from build123d import *

# Parameters (mm, degrees)
BASE_DEPTH            = 7.5
MOUNT_START           = -2
MOUNT_DEPTH           = 4
MOUNT_HOLE_DEPTH      = 204.131478566
MOUNT_HOLE_DEPTH_BACK = 204.131478566
SKETCH12_R            = 1.5
SKETCH14_R            = 1.5
SHAFT_HOLE_DEPTH      = 37.394984425
SKETCH13_W            = 2.5
SKETCH13_H            = 3


with BuildPart() as part:
    # Sketch9 → base (new, symmetric)
    with BuildSketch(Plane(origin=(0, 0, 0), x_dir=(1, 0, 0), z_dir=(0, 1, 0))):
        with BuildLine():
            ThreePointArc((-187.113473072, -32.993153757), (-190, 0), (-187.113473072, 32.993153757))
            Line((-187.113473072, 32.993153757), (-196.961550602, 34.729635533))
            ThreePointArc((-196.961550602, 34.729635533), (-200, 0), (-196.961550602, -34.729635533))
            Line((-196.961550602, -34.729635533), (-187.113473072, -32.993153757))
        make_face()
    extrude(amount=BASE_DEPTH, both=True)

    # Sketch11 → mount (cut)
    with BuildSketch(Plane(origin=(0, 0, 0), x_dir=(1, 0, 0), z_dir=(0, 1, 0)).offset(MOUNT_START)):
        with BuildLine():
            Line((-189.73665961, -10), (-199.749843554, -10))
            ThreePointArc((-199.749843554, -10), (-198.7407137, -22.408228804), (-196.961550602, -34.729635533))
            Line((-196.961550602, -34.729635533), (-187.113473072, -32.993153757))
            ThreePointArc((-187.113473072, -32.993153757), (-188.775466906, -21.536552519), (-189.73665961, -10))
        make_face()
        with BuildLine():
            Line((-189.73665961, 10), (-199.749843554, 10))
            ThreePointArc((-199.749843554, 10), (-198.7407137, 22.408228804), (-196.961550602, 34.729635533))
            Line((-196.961550602, 34.729635533), (-187.113473072, 32.993153757))
            ThreePointArc((-187.113473072, 32.993153757), (-188.775466906, 21.536552519), (-189.73665961, 10))
        make_face()
    extrude(amount=MOUNT_DEPTH, mode=Mode.SUBTRACT)

    # Sketch12 → mount hole (cut, two sides: drawn at the far end of the back side and taken through both)
    with BuildSketch(Plane(origin=(0, 0, 0), x_dir=(1, 0, 0), z_dir=(0, 1, 0)).offset(-MOUNT_HOLE_DEPTH_BACK)):
        with Locations(Location((-193.331747968, 25.452607483, 0), (0, 0, 270))):
            Circle(SKETCH12_R)
        with Locations(Location((-194.257966128, 16.995369836, 0), (0, 0, 270))):
            Circle(SKETCH12_R)
        with Locations(Location((-194.257966128, -16.995369836, 0), (0, 0, 270))):
            Circle(SKETCH12_R)
        with Locations(Location((-193.331747968, -25.452607483, 0), (0, 0, 270))):
            Circle(SKETCH12_R)
    extrude(amount=MOUNT_HOLE_DEPTH + MOUNT_HOLE_DEPTH_BACK, mode=Mode.SUBTRACT)

    # Sketch14 → shaft hole (cut, through all)
    with BuildSketch(Plane.ZY.offset(195)):
        Circle(SKETCH14_R)
    extrude(amount=-SHAFT_HOLE_DEPTH, mode=Mode.SUBTRACT)

    # Sketch13 → bearing hole (revolve, cut)
    with BuildSketch(Plane(origin=(0, 0, 0), x_dir=(1, 0, 0), z_dir=(0, 1, 0)), mode=Mode.PRIVATE) as bearing_hole_sk:
        with Locations((-195, 1.5)):
            Rectangle(SKETCH13_W, SKETCH13_H)
    revolve(bearing_hole_sk.sketch.rotate(Axis((0, 0, 0), (-1, 0, 0)), 180), axis=Axis((0, 0, 0), (-1, 0, 0)), mode=Mode.SUBTRACT)


solid = part.part
Source: CAD feature listing. Evaluate the final solid. Frame: model axes, mm. A direction names the side the tool comes from. Give positions to 0.01 mm unless a question says otherwise; leave off trailing zeros. Order: outer loops, then holes, each group sorted by start corner. A loop starts at its lowest first (then second) coordinate and runs counter-clockwise, first axis right, second up. Notation, with made-up numbers: (45.25, 33.25) -> (61.25, 33.25) arc R13 ccw to (61.25, 37.25) -> close; hole circle Ø4 at (69.25, 20). An arc over 180 degrees is marked (long way). Write item = value, one per line.
Item 1: Section query D-D (z = 0). Output: boundary loops of the cut face in (x, y).
Check result:
outline = (-200, -7.5) -> (-190, -7.5) -> (-190, -1.5) -> (-193.75, -1.5) -> (-193.75, -3) -> (-196.25, -3) -> (-196.25, 3) -> (-193.75, 3) -> (-193.75, 1.5) -> (-190, 1.5) -> (-190, 7.5) -> (-200, 7.5) -> close
Item 2: Section query A-A (z = 26). Output: boundary loops of the cut face in (x, y), then the cut area to 3 significant figures.
Check result:
outline = (-198.3, -7.5) -> (-194.73, -7.5) -> (-194.73, -2) -> (-198.3, -2) -> close; (-198.3, 2) -> (-194.73, 2) -> (-194.73, 7.5) -> (-198.3, 7.5) -> close; (-191.94, -7.5) -> (-188.21, -7.5) -> (-188.21, -2) -> (-191.94, -2) -> close; (-191.94, 2) -> (-188.21, 2) -> (-188.21, 7.5) -> (-191.94, 7.5) -> close
area = 80.3 mm²
Item 3: Set-up query: faces 1 (the face through (-193, 2, -23)), 2 (the face through (-194, -2, 22)), 3 (the face through (-191.9, 0.07, -1.5)), 4 (the face through (-196.25, 0, 0)). Return all of +Z, -Z, +X, -X, +Y, -Y with unobstructed straight access to the full face (end or side cutting, diameter ignored); none if empty.
Check result:
face_1 = -Z, +X, -X
face_2 = +Z, +X, -X
face_3 = +X
face_4 = none
Item 4: Mould query, pull axis Z, two halves, no side actions, for faces 5 (the face through (-194.796, 4.712, 25.127)), 6 (the face through (-192.77, -4.79, 16.8)), 7 (the face through (-194, 2, 22)), 8 (the face through (-191.97, 4.79, -33.85)). Classes: +Z half, -Z half, draft (parallel to the pull), parting line (faces both ways), or undercut.
Check result:
face_5 = undercut
face_6 = undercut
face_7 = draft
face_8 = -Z half
Item 5: Section query C-C (y = 0). Output: boundary loops of the cut face in (x, z).
Check result:
outline = (-199.75, -10) -> (-189.74, -10) arc R190 cw to (-189.99, -1.5) -> (-193.75, -1.5) -> (-193.75, -3) -> (-196.25, -3) -> (-196.25, 3) -> (-193.75, 3) -> (-193.75, 1.5) -> (-189.99, 1.5) arc R190 cw to (-189.74, 10) -> (-199.75, 10) arc R200 ccw to start
Item 6: Ray query, probe 1 along Y at (x, z) = (-197, 28.5); probe 2 along Z at (x, y) = (-193.25, -3); probe 3 along Z at (x, y) = (-193, 3.25). Return the intervals inside material, ascending.
Check result:
probe_1 = -7.5 to -2, 2 to 7.5
probe_2 = -34.08 to -26.95, -23.95 to -18.11, -15.88 to 15.88, 18.11 to 23.95, 26.95 to 34.08
probe_3 = -34.03 to -26.92, -23.99 to -17.81, -16.18 to 16.18, 17.81 to 23.99, 26.92 to 34.03
Item 7: Section query B-B (x = -191.25). Output: boundary loops of the cut face in (y, z), then the cut area to 3 significant figures.
Check result:
outline = (-7.5, -33.72) -> (-2, -33.72) -> (-2, -10) -> (2, -10) -> (2, -33.72) -> (7.5, -33.72) -> (7.5, 33.72) -> (2, 33.72) -> (2, 10) -> (-2, 10) -> (-2, 33.72) -> (-7.5, 33.72) -> close; hole circle Ø3 at (0, 0)
area = 815 mm²
Item 8: Contact query for flat-ended pins moving along their axis: pin 1 (1.5 mm diameter, centred on y = -1, z = -5, fed in from +X); pin 2 (3 mm diameter, centred on y = -3.5, z = -11, fed in from +X); pin 3 (2.5 mm diameter, centred on x = -193.33, z = -25.45, fed in from -Y); pin 4 (8 mm diameter, centred on y = 5, z = -16, fed in from +X). Output: stop coordinate, or through.
Check result:
pin_1 = -189.91
pin_2 = -189.59
pin_3 = through
pin_4 = -188.94
